```python
from build123d import *

# Parameters (mm, degrees)
ESQUISSE1_R             = 25
ESQUISSE1_R_2           = 5.1
BOSS_EXTRU_1_DEPTH      = 7
ESQUISSE2_R             = 25
ESQUISSE2_R_2           = 3
BOSS_EXTRU_2_DEPTH      = 3
BOSS_EXTRU_3_DEPTH      = 8.5
BOSS_EXTRU_3_DEPTH_BACK = 7
ESQUISSE3_R             = 27
ESQUISSE3_R_2           = 25


with BuildPart() as part:
    # Esquisse1 → Boss.-Extru.1 (new body)
    with BuildSketch(Plane(origin=(0, 0, 0), x_dir=(1, 0, 0), z_dir=(0, 1, 0))):
        with Locations(Location((0, 0, 0), (0, 0, 270))):
            Circle(ESQUISSE1_R)
        with Locations(Location((0, 0, 0), (0, 0, 270))):
            Circle(ESQUISSE1_R_2, mode=Mode.SUBTRACT)
    extrude(amount=BOSS_EXTRU_1_DEPTH)

    # Esquisse2 → Boss.-Extru.2 (add)
    with BuildSketch(Plane.XZ):
        with Locations(Location((0, 0, 0), (0, 0, 90))):
            Circle(ESQUISSE2_R)
        with Locations(Location((0, 0, 0), (0, 0, 270))):
            Circle(ESQUISSE2_R_2, mode=Mode.SUBTRACT)
    extrude(amount=-BOSS_EXTRU_2_DEPTH)

    # Esquisse3 → Boss.-Extru.3 (add, two sides: drawn at the far end of the back side and taken through both)
    with BuildSketch(Plane(origin=(0, 7, 0), x_dir=(1, 0, 0), z_dir=(0, 1, 0)).offset(-BOSS_EXTRU_3_DEPTH_BACK)):
        with Locations(Location((0, 0, 0), (0, 0, 270))):
            Circle(ESQUISSE3_R)
        with Locations(Location((0, 0, 0), (0, 0, 270))):
            Circle(ESQUISSE3_R_2, mode=Mode.SUBTRACT)
    extrude(amount=BOSS_EXTRU_3_DEPTH + BOSS_EXTRU_3_DEPTH_BACK)


solid = part.part
```
Design review of the part built by this model. Coordinates are the model's own, in mm. A direction names the side the tool comes from. Coordinates: 2 decimals unless noted, no trailing zeros. Order: outer loops, then holes, each group sorted by start corner. A loop starts at its lowest first (then second) coordinate and runs counter-clockwise, first axis right, second up. Notation, with made-up numbers: M 11.25,-7.75 L 51.25,-7.75 A29 cw 51.25,31.25 Z; hole C -8,3 d5. An arc over 180 degrees is marked long. Answer as a JSON object with one key per item and string values. Group by question number.
1) Add section C-C, the plane y = 5.75. Write out the cut boundary in (x, z), then the cut area to 3 significant figures.
2) Add section B-B, the plane z = 0. Write out the cut boundary in (x, y).
3) Add section A-A, the plane x = 0. Write out the cut boundary in (y, z), then the cut area to 3 significant figures.
4) Wall thickness on L1, parallel to X at y = 1.1, z = 0; L2, parallel to X at y = 11.75, z = 0; L3, parallel to Y at x = 8.5, z = 3: over which ranges is each line inside the solid? List them lowest first.
5) Tool access review of faces 4 (the cylindrical face through (1.532, 4.972, 4.864)), 5 (the cylindrical face through (0.9, 1.48, -2.86)): name each direction out of +Z, -Z, +X, -X, +Y, -Y from which nothing blocks a thin tool from reaching the whole face with its end or side.
6) For pin 1 (6 mm diameter, centred on x = 5, y = 14, fed in from +Z); pin 2 (2 mm diameter, centred on y = 5.5, z = 11, fed in from +X); pin 3 (11 mm diameter, centred on x = 0, z = 2, fed in from +Y), all flat-tipped, find the tip position at first contact; note any pin that passes through.
7) Mouldability with a two-part tool opening along Z and no side actions: class faces 1 (the flat face through (-8, 15.5, 24)), 2 (the cylindrical face through (-26.36, 7.64, -5.85)), 3 (the cylindrical face through (7.509, 11.19, 23.846)) as pulls with the +Z half, pulls with the -Z half, needs draft (parallel to the pull), parting line crosses it, or undercut.
8) Add section D-D, the plane z = -19. Write out the cut boundary in (x, y).
Computed values:
{
 "1": {"outline": "C 0,0 d54; hole C 0,0 d10.2", "area": "2,210 mm^2"},
 "2": {"outline": "M -27,0 L -3,0 L -3,3 L -5.1,3 L -5.1,7 L -25,7 L -25,15.5 L -27,15.5 Z; M 3,0 L 27,0 L 27,15.5 L 25,15.5 L 25,7 L 5.1,7 L 5.1,3 L 3,3 Z"},
 "3": {"outline": "M 0,-27 L 15.5,-27 L 15.5,-25 L 7,-25 L 7,-5.1 L 3,-5.1 L 3,-3 L 0,-3 Z; M 0,3 L 3,3 L 3,5.1 L 7,5.1 L 7,25 L 15.5,25 L 15.5,27 L 0,27 Z", "area": "353 mm^2"},
 "4": {"L1": "x = -27 to -3, 3 to 27", "L2": "x = -27 to -25, 25 to 27", "L3": "y = 0 to 7"},
 "5": {"face 4": "+Y", "face 5": "+Y, -Y"},
 "6": {"pin 1": "stops at z = 26.93", "pin 2": "stops at x = 25.08", "pin 3": "stops at y = 7"},
 "7": {"face 1": "needs draft", "face 2": "parting line crosses it", "face 3": "undercut"},
 "8": {"outline": "M -19.18,0 L 19.18,0 L 19.18,15.5 L 16.25,15.5 L 16.25,7 L -16.25,7 L -16.25,15.5 L -19.18,15.5 Z"}
}
